from build123d import *

# Parameters (mm, degrees)
F0_R     = 25
F1_DEPTH = 4
F3_DEPTH = 73


# Not quite as in the source:
# - an extrude ends at something that could not be found from the text; its depth is read off the source's solid


with BuildPart() as f1:
    # F0 (on Top) → F1 (new body)
    with BuildSketch(Plane.XY):
        Circle(F0_R)
    extrude(amount=F1_DEPTH)

    # F2 (on face) → F3 (cut, through all)
    with BuildSketch(Plane.XY.offset(4)):
        with BuildLine():
            Line((-3, -25), (0, -25))
            ThreePointArc((0, -25), (-1.5027171558, -24.9547959549), (-3, -24.819347292))
            Line((-3, -24.819347292), (-3, -25))
        make_face()
        with BuildLine():
            Line((0, -25), (0, -15))
            Line((0, -15), (-3, -15))
            Line((-3, -15), (-3, -24.819347292))
            ThreePointArc((-3, -24.819347292), (-1.5027171558, -24.9547959549), (0, -25))
        make_face()
    extrude(amount=-F3_DEPTH, mode=Mode.SUBTRACT)


solid = f1.part
Can you work these out from the model? Positions are in its coordinate system, mm. A direction names the side the tool comes from. Give positions to 0.01 mm unless a question says otherwise; leave off trailing zeros. Write each loop counter-clockwise with the first axis right and the second up, starting at its lowest first coordinate (ties: lowest second). Pieces come first, ordered by that corner, then holes. Notation, with made-up numbers: (56.25, 28) -> (80.25, 28) arc R8 cw to (80.25, 36) -> close; hole circle Ø8 at (10, -13.5). An arc over 180 degrees is marked (long way). Answer as a JSON object with one key per item and string values. Group by question number.
Item 1: Suppose I cut it at B-B (y = -8). Please give me the cut outline in (x, z), plus the area to 3 significant figures.
Item 2: Please list where these lines run through material, in increasing order: line 1 (X direction, y = -15.5, z = 2.5); line 2 (Y direction, x = -0.5, z = 2.6) (3 decimals); line 3 (X direction, y = -16, z = 2.9). Write a range as [from, to].
Item 3: For faces 3 (the face through (-3, -20, 2)), 4 (the face through (0, 0, 0)), which set-ups out of +Z, -Z, +X, -X, +Y, -Y let a thin tool reach every point of the face, with its end or its side?
Item 4: We'd pull the mould along X, two halves only. Please class faces 1 (the face through (0, -20, 2)), 2 (the face through (0, 0, 4)): +X half, -X half, draft (parallel to the pull), parting line (faces both ways), or undercut.
Item 5: I'm going to push flat-ended pins straight in: P1, Ø1.5, axis at x = -1.5, z = 2.5, coming from the -Y side; P2, Ø1.5, axis at x = -20, z = 1.5, coming from the -Y side. Where does each tip first touch, or does it pass through?
Item 6: Suppose I cut it at A-A (z = 1.15). Please give me the cut outline in (x, y).
Findings:
{
 "1": {"outline": "(-23.69, 0) -> (23.69, 0) -> (23.69, 4) -> (-23.69, 4) -> close", "area": "189 mm²"},
 "2": {"line 1": "x = [-19.62, -3], [0, 19.62]", "line 2": "y = [-15, 24.995]", "line 3": "x = [-19.21, -3], [0, 19.21]"},
 "3": {"face 3": "+Z, -Z, -Y", "face 4": "-Z, +X, -X, +Y, -Y"},
 "4": {"face 1": "undercut", "face 2": "draft"},
 "5": {"P1": "stops at y = -15", "P2": "stops at y = -15.95"},
 "6": {"outline": "(-3, -24.82) -> (-3, -15) -> (0, -15) -> (0, -25) arc R25 ccw (long way) to start"}
}
